```python
from build123d import *

# Parameters (mm, degrees)
F0_W     = 30
F0_H     = 75
F1_DEPTH = 40
F2_W     = 5
F2_H     = 10
F3_DEPTH = 30.001


with BuildPart() as f1:
    # F0 (on Top) → F1 (new body)
    with BuildSketch(Plane.XY):
        Rectangle(F0_W, F0_H)
    extrude(amount=F1_DEPTH)

    # F2 (on face) → F3 (cut, through all)
    with BuildSketch(Plane.YZ.offset(15)):
        with Locations((-35, 20)):
            Rectangle(F2_W, F2_H)
        with Locations((35, 20)):
            Rectangle(F2_W, F2_H)
        Polygon((-2.5, 20), (-2.5, 15), (2.5, 15), (2.5, 20), (27.5, 40), (-27.5, 40), align=None)
    extrude(amount=-F3_DEPTH, mode=Mode.SUBTRACT)


solid = f1.part
```
Geometry check sheet. Reference: the model listing, model coordinates, mm. A direction names the side the tool comes from. Round coordinates to 2 decimals unless told otherwise and drop trailing zeros. Loops run counter-clockwise (first coordinate to the right, second up) from the corner with the lowest first, then second, coordinate; pieces in that order, holes last. Notation, with made-up numbers: M 61.25,21.25 L 81.25,21.25 A20 cw 81.25,37.25 Z; hole C 25,65 d7. An arc over 180 degrees is marked long. Return JSON: item names as keys, results as strings. Group by question number.
(1) Section check A-A, the plane z = 31. Enter the section's corners in (x, y).
(2) Section check D-D, the plane y = -18.5. Enter the section's corners in (x, z).
(3) Go/stop test with flat-tipped pins: pin 1 (3 mm diameter, centred on x = 0.5, y = 2.5, fed in from +Z); pin 2 (5 mm diameter, centred on x = 3, z = 22, fed in from -Y); pin 3 (12 mm diameter, centred on x = 9, y = 1.5, fed in from +Z). Record where each tip stops, or that it passes through.
(4) Scan lines: line 1 along Z through (x, y) = (3.25, -34); line 2 along Y through (x, z) = (11, 29); line 3 along Y through (x, z) = (4.5, 29.5) (3 decimals). Record each from-to range of solid material in increasing order. Write a range as [from, to].
(5) Mould release check, pull along Y, two halves, no side actions. Record for faces 5 (the face through (0, 15, 30)), 6 (the face through (-15, -1, 11)), 7 (the face through (0, -15, 30)), 8 (the face through (0, -32.5, 20)): pulls with the +Y half, pulls with the -Y half, needs draft (parallel to the pull), parting line crosses it, or undercut.
(6) Section check C-C, the plane y = -1. Enter the section's corners in (x, z), and give its area (3 significant figures).
(7) Section check B-B, the plane x = -12.5. Enter the section's corners in (y, z).
(8) Set-up check for faces 1 (the face through (0, 37.5, 32)), 2 (the face through (0, -2.5, 18)), 3 (the face through (0, -35, 15)), 4 (the face through (0, 32.5, 20)): record each of +Z, -Z, +X, -X, +Y, -Y from which the full face is reachable in a straight line by a thin tool's end or side.
Data:
{
 "1": {"outline": "M -15,-37.5 L 15,-37.5 L 15,-16.25 L -15,-16.25 Z; M -15,16.25 L 15,16.25 L 15,37.5 L -15,37.5 Z"},
 "2": {"outline": "M -15,0 L 15,0 L 15,32.8 L -15,32.8 Z"},
 "3": {"pin 1": "z = 21.2", "pin 2": "y = -32.5", "pin 3": "z = 24"},
 "4": {"line 1": "[0, 15], [25, 40]", "line 2": "[-37.5, -13.75], [13.75, 37.5]", "line 3": "[-37.5, -14.375], [14.375, 37.5]"},
 "5": {"face 5": "undercut", "face 6": "needs draft", "face 7": "undercut", "face 8": "pulls with the -Y half"},
 "6": {"outline": "M -15,0 L 15,0 L 15,15 L -15,15 Z", "area": "450 mm²"},
 "7": {"outline": "M -37.5,0 L 37.5,0 L 37.5,15 L 32.5,15 L 32.5,25 L 37.5,25 L 37.5,40 L 27.5,40 L 2.5,20 L 2.5,15 L -2.5,15 L -2.5,20 L -27.5,40 L -37.5,40 L -37.5,25 L -32.5,25 L -32.5,15 L -37.5,15 Z"},
 "8": {"face 1": "+Z, -Z, +X, -X, +Y", "face 2": "+Z, +X, -X", "face 3": "+X, -X, -Y", "face 4": "+X, -X, +Y"}
}
